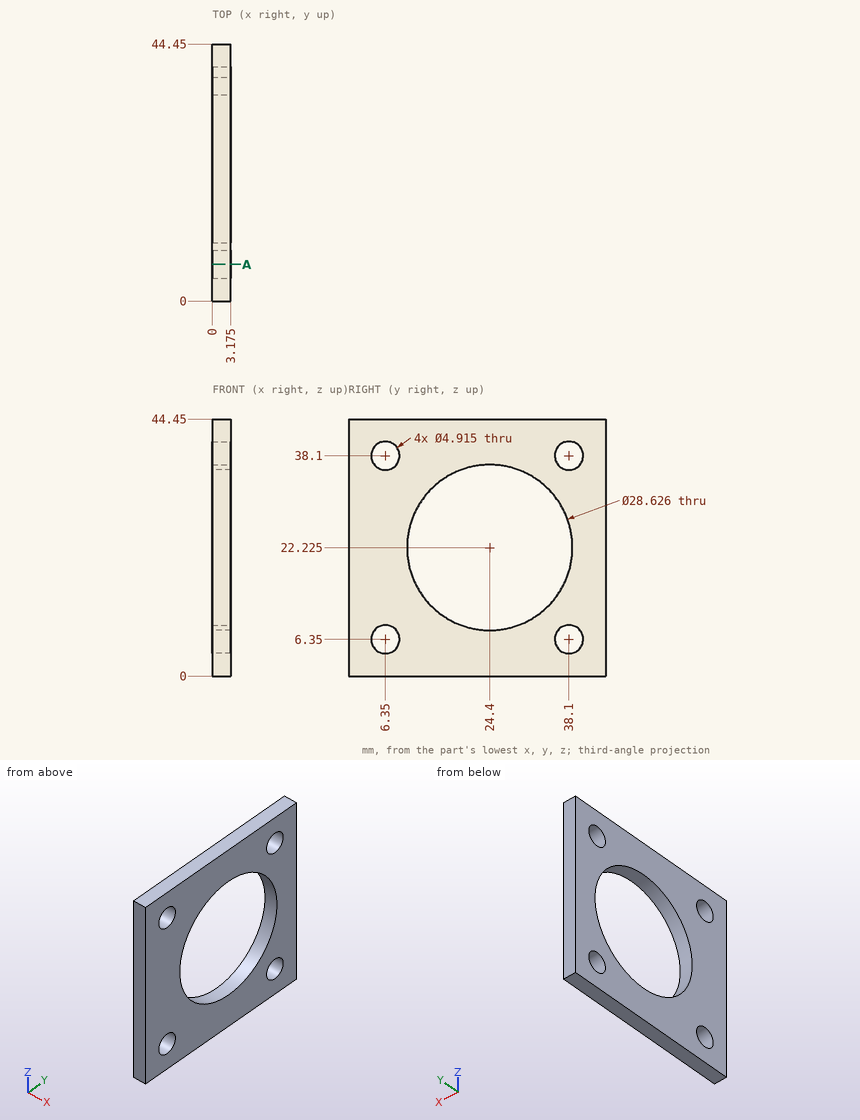
Could you check a few things on this drawing? It's one solid part, dimensions in mm from its lowest x, y, z. Give positions to 0.01 mm unless a question says otherwise; leave off trailing zeros. Answer as a JSON object with one key per item and string values.
Q1. Please list where these lines run through material, in increasing order: L1, parallel to Y at x = 1.9, z = 38.1; L2, parallel to Y at x = 2.2, z = 5.5; L3, parallel to Z at x = 2.5, y = 4.5.
Taken from the geometry:
{"L1": "y = 0 to 3.89, 8.81 to 35.64, 40.56 to 44.45", "L2": "y = 0 to 4.04, 8.66 to 35.79, 40.41 to 44.45", "L3": "z = 0 to 4.73, 7.97 to 36.48, 39.72 to 44.45"}
Q2. Will this pin go through, and if not, where does the flat tip stop? pin 1 Ø12 at (y, z) = (35, 19.5) entering from +X (3 decimals).
Taken from the geometry:
{"pin 1": "stops at x = 3.175"}
Q3. Suppose I cut it at A-A on y = 6.35. Count the separate pieces of the cut face and the enclosed holes in it, then the cut area to 3 significant figures.
Taken from the geometry:
{"separate pieces": "3", "enclosed holes": "0", "area": "110 mm²"}
